Here's the drawing with two shaded views (mm, measured from the low corner). I have some questions. A direction names the side the tool comes from. Coordinates: 2 decimals unless noted, no trailing zeros. Order: outer loops, then holes, each group sorted by start corner. A loop starts at its lowest first (then second) coordinate and runs counter-clockwise, first axis right, second up. Notation, with made-up numbers: (3.25, -6.5) - (49.25, -6.5) arc R21 cw to (49.25, 14.5) - close; hole circle Ø3 at (23, 74.5). An arc over 180 degrees is marked (long way). Answer as CSV lines item,"result". Start each with the question number.
1. I want a section at C-C, the plane y = 6. List the corners of the cut face in (x, z) for me, and give its area (3 significant figures).
2. I want a section at D-D, the plane z = 1. List the corners of the cut face in (x, y) for me.
3. I need wall thicknesses on probe 1 along Z at (x, y) = (4.25, 6.5); probe 2 along Y at (x, z) = (11.25, 11.25). Which ranges of each line are inside material? Lowest first, please.
4. For pin 1 (6 mm diameter, centred on x = 8.5, z = 6.5, fed in from +Y), with a flat end and sliding along its axis, tell me the tip position at first contact or that it passes through.
5. I want a section at B-B, the plane x = 10. List the corners of the cut face in (y, z) for me, and give its area (3 significant figures).
6. I want a section at A-A, the plane y = 1.5. List the corners of the cut face in (x, z) for me.
7. Thinking about a two-plate mould opening in X: for the marked faces 3, 4 and 5, which applies, released by +X, released by -X, zero draft, split by the parting line, or undercut?
8. For the marked faces 1 and 2, which set-ups out of +Z, -Z, +X, -X, +Y, -Y let a thin tool reach every point of the face, with its end or its side?
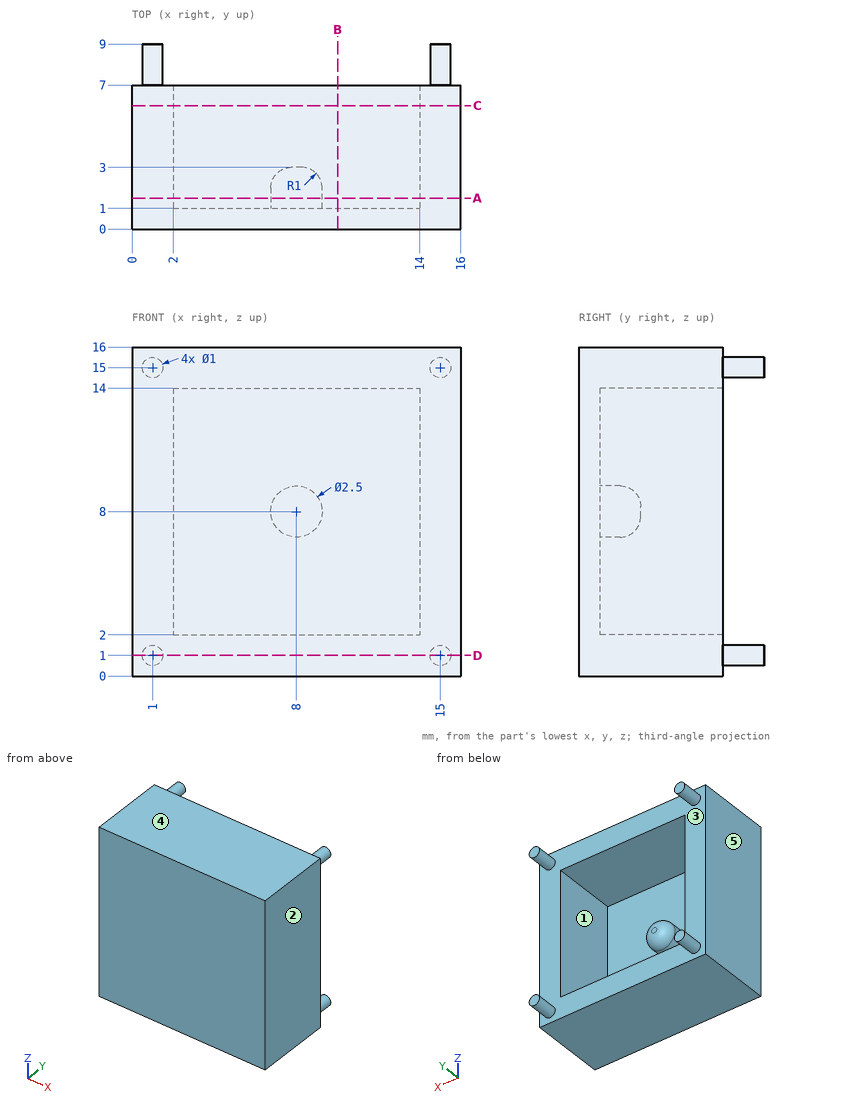
Solved:
1,outline,"(0, 0) - (16, 0) - (16, 16) - (0, 16) - close; hole (2, 2) - (14, 2) - (14, 14) - (2, 14) - close"
1,area,"112 mm2"
2,outline,"(0, 0) - (16, 0) - (16, 7) - (15.5, 7) - (15.5, 9) - (14.5, 9) - (14.5, 7) - (1.5, 7) - (1.5, 9) - (0.5, 9) - (0.5, 7) - (0, 7) - close"
3,probe 1,"z = 0 to 2, 14 to 16"
3,probe 2,"y = 0 to 1"
4,pin 1,"stops at y = 3"
5,outline,"(0, 0) - (7, 0) - (7, 2) - (1, 2) - (1, 14) - (7, 14) - (7, 16) - (0, 16) - close"
5,area,"40.0 mm2"
6,outline,"(0, 0) - (16, 0) - (16, 16) - (0, 16) - close; circle Ø2.5 at (8, 8); hole (2, 2) - (14, 2) - (14, 14) - (2, 14) - close"
7,face 3,"undercut"
7,face 4,"zero draft"
7,face 5,"released by -X"
8,face 1,"+Y"
8,face 2,"+Z, -Z, +X, +Y, -Y"
